Can you work these out from the model? Positions are in its coordinate system, mm. Coordinates: 2 decimals unless noted, no trailing zeros. Order: outer loops, then holes, each group sorted by start corner. A loop starts at its lowest first (then second) coordinate and runs counter-clockwise, first axis right, second up. Notation, with made-up numbers: (-8.75, -30) -> (27.25, -30) arc R37 ccw to (27.25, 6) -> close; hole circle Ø5 at (38.25, 78). An arc over 180 degrees is marked (long way). Return JSON: item names as keys, results as strings. Group by question number.
1) If we section it at A-A, the plane y = 0: Please give me the cut outline in (x, z).
2) If I drill on probe 1 along Y at (x, z) = (0, 105); probe 2 along Y at (x, z) = (6, 127); probe 3 along X at (y, z) = (7.5, 106.5), over which ranges is the centre line in solid material (lowest first)? Write a range as from..to.
3) For pin 1 (3 mm diameter, centred on x = 0.5, z = 111.5, fed in from -Y); pin 2 (1.1 mm diameter, centred on x = -0.5, z = 114, fed in from +Y); pin 3 (3 mm diameter, centred on y = -0.5, z = 75.5, fed in from -X), each with a flat end and sliding along its axis, tell me the tip position at first contact or that it passes through.
Autodesk Inventor part; units mm, degrees
ref_plane "Start Plane" through (0, 0, 10.031) normal (0, 0, 1) x (1, 0, 0)
ref_plane "End Plane" through (0, 0, 150) normal (0, 0, 1) x (1, 0, 0)
ref_plane "Work Plane6" through (-400, 9, 10.031) normal (0, 0, -1) x (-1, 0, 0)
ref_plane "Start Plane" through (0, 0, 10.031) normal (0, 0, 1) x (1, 0, 0)
ref_plane "End Plane" through (0, 0, 150) normal (0, 0, 1) x (1, 0, 0)
sketch "Sketch" plane through (0, 0, 0) normal (0, 0, 1) x (1, 0, 0)
  line L0 (0, 0) -> (2.5, 0) construction
  line L1 (0, 0) -> (0, 2.5) construction
  line L2 (0, 4) -> (0, -4) construction
  line L3 (0, 4) -> (1.7574, 4)
  arc A0 (1.7574, 4) -> (3.1716, 4.5858) centre (1.7574, 6) ccw
  line L4 (3.1716, 4.5858) -> (5.7322, 7.1464)
  line L5 (-4, 0) -> (4, 0) construction
  line L6 (4, 0) -> (4, 1.7574)
  arc A1 (4.5858, 3.1716) -> (4, 1.7574) centre (6, 1.7574) ccw
  line L7 (4.5858, 3.1716) -> (7.1464, 5.7322)
  line L8 (0, 0) -> (10, 10) construction
  line L9 (0, 0) -> (19.6827, 0) construction
  arc A2 (8, 5.3787) -> (7.1464, 5.7322) centre (7.5, 5.3787) ccw
  line L10 (8, 5.3787) -> (8, 3.5)
  arc A3 (8, 3.5) -> (8.5, 3) centre (8.5, 3.5) ccw
  line L11 (8.5, 3) -> (9.5, 3)
  arc A4 (9.5, 3) -> (10, 3.5) centre (9.5, 3.5) ccw
  line L12 (10, 3.5) -> (10, 9)
  line L13 (10, 9) -> (10, 10) construction
  arc A5 (5.7322, 7.1464) -> (5.3787, 8) centre (5.3787, 7.5) ccw
  line L14 (5.3787, 8) -> (3.5, 8)
  arc A6 (3, 8.5) -> (3.5, 8) centre (3.5, 8.5) ccw
  line L15 (3, 8.5) -> (3, 9.5)
  arc A7 (3.5, 10) -> (3, 9.5) centre (3.5, 9.5) ccw
  line L16 (3.5, 10) -> (9, 10)
  arc A8 (10, 9) -> (9, 10) centre (9, 9) ccw
  line L17 (0, 4) -> (-1.7574, 4)
  arc A9 (-3.1716, 4.5858) -> (-1.7574, 4) centre (-1.7574, 6) ccw
  line L18 (-3.1716, 4.5858) -> (-5.7322, 7.1464)
  line L19 (-4, 0) -> (-4, 1.7574)
  arc A10 (-4, 1.7574) -> (-4.5858, 3.1716) centre (-6, 1.7574) ccw
  line L20 (-4.5858, 3.1716) -> (-7.1464, 5.7322)
  arc A11 (-7.1464, 5.7322) -> (-8, 5.3787) centre (-7.5, 5.3787) ccw
  line L21 (-8, 5.3787) -> (-8, 3.5)
  arc A12 (-8.5, 3) -> (-8, 3.5) centre (-8.5, 3.5) ccw
  line L22 (-8.5, 3) -> (-9.5, 3)
  arc A13 (-10, 3.5) -> (-9.5, 3) centre (-9.5, 3.5) ccw
  line L23 (-10, 3.5) -> (-10, 9)
  arc A14 (-5.3787, 8) -> (-5.7322, 7.1464) centre (-5.3787, 7.5) ccw
  line L24 (-5.3787, 8) -> (-3.5, 8)
  arc A15 (-3.5, 8) -> (-3, 8.5) centre (-3.5, 8.5) ccw
  line L25 (-3, 8.5) -> (-3, 9.5)
  arc A16 (-3, 9.5) -> (-3.5, 10) centre (-3.5, 9.5) ccw
  line L26 (-3.5, 10) -> (-9, 10)
  arc A17 (-9, 10) -> (-10, 9) centre (-9, 9) ccw
  line L27 (0, -4) -> (-1.7574, -4)
  arc A18 (-1.7574, -4) -> (-3.1716, -4.5858) centre (-1.7574, -6) ccw
  line L28 (-3.1716, -4.5858) -> (-5.7322, -7.1464)
  arc A19 (-5.7322, -7.1464) -> (-5.3787, -8) centre (-5.3787, -7.5) ccw
  line L29 (-5.3787, -8) -> (-3.5, -8)
  arc A20 (-3, -8.5) -> (-3.5, -8) centre (-3.5, -8.5) ccw
  line L30 (-3, -8.5) -> (-3, -9.5)
  arc A21 (-3.5, -10) -> (-3, -9.5) centre (-3.5, -9.5) ccw
  line L31 (-3.5, -10) -> (-9, -10)
  arc A22 (-10, -9) -> (-9, -10) centre (-9, -9) ccw
  line L32 (-10, -3.5) -> (-10, -9)
  arc A23 (-9.5, -3) -> (-10, -3.5) centre (-9.5, -3.5) ccw
  line L33 (-8.5, -3) -> (-9.5, -3)
  arc A24 (-8, -3.5) -> (-8.5, -3) centre (-8.5, -3.5) ccw
  line L34 (-8, -5.3787) -> (-8, -3.5)
  arc A25 (-8, -5.3787) -> (-7.1464, -5.7322) centre (-7.5, -5.3787) ccw
  line L35 (-4.5858, -3.1716) -> (-7.1464, -5.7322)
  arc A26 (-4.5858, -3.1716) -> (-4, -1.7574) centre (-6, -1.7574) ccw
  line L36 (-4, 0) -> (-4, -1.7574)
  line L37 (3.5, -10) -> (9, -10)
  arc A27 (9, -10) -> (10, -9) centre (9, -9) ccw
  line L38 (10, -3.5) -> (10, -9)
  arc A28 (10, -3.5) -> (9.5, -3) centre (9.5, -3.5) ccw
  line L39 (8.5, -3) -> (9.5, -3)
  arc A29 (8.5, -3) -> (8, -3.5) centre (8.5, -3.5) ccw
  line L40 (8, -5.3787) -> (8, -3.5)
  arc A30 (7.1464, -5.7322) -> (8, -5.3787) centre (7.5, -5.3787) ccw
  line L41 (4.5858, -3.1716) -> (7.1464, -5.7322)
  arc A31 (4, -1.7574) -> (4.5858, -3.1716) centre (6, -1.7574) ccw
  line L42 (4, 0) -> (4, -1.7574)
  line L43 (5.3787, -8) -> (3.5, -8)
  arc A32 (5.3787, -8) -> (5.7322, -7.1464) centre (5.3787, -7.5) ccw
  line L44 (3.1716, -4.5858) -> (5.7322, -7.1464)
  arc A33 (3.1716, -4.5858) -> (1.7574, -4) centre (1.7574, -6) ccw
  line L45 (0, -4) -> (1.7574, -4)
  arc A34 (3.5, -8) -> (3, -8.5) centre (3.5, -8.5) ccw
  line L46 (3, -8.5) -> (3, -9.5)
  arc A35 (3, -9.5) -> (3.5, -10) centre (3.5, -9.5) ccw
  circle A36 centre (0, 0) radius 2.5
  dimension "d1" = 8
  dimension "d2" = 2
  dimension "d3" = 8
  dimension "d4" = 2
  dimension "d5" = 2
  dimension "d7" = 45
  dimension "d8" = 0.5
  dimension "d9" = 0.5
  dimension "d10" = 0.5
  dimension "d12" = 2
  dimension "d17" = 7
  dimension "d18" = 10
  dimension "d19" = 0.5
  dimension "d20" = 1
  dimension "d21" = 0.5
  dimension "d22" = 0.5
  dimension "d23" = 2
  dimension "d24" = 7
  dimension "d25" = 5
extrude "Body" add sketch "Sketch" along normal up to surface (139.969 mm away) from surface at 10.031
sketch "Sketch6" plane through (0, 0, 0) normal (0, 0, 1) x (1, 0, 0)
  line L0 (0, 0) -> (10, 0)
ref_plane "Work Plane5" through (0, 0, 0) normal (0, -1, 0) x (1, 0, 0)
sketch "Sketch7" plane through (0, 0, 0) normal (0, -1, 0) x (1, 0, 0)
  line L0 (-2, 10.031) -> (12, 10.031)
  line L1 (-2, 150) -> (12, 150)
  dimension "d33" = 139.969
ref_plane "Work Plane6" through (-400, 9, 10.031) normal (0, 0, -1) x (-1, 0, 0)
split "Split1" plane through (-400, 9, 10.031) removes the side toward (0, 0, -1)
equation "\"d1\" = 0.8 * sigma"
equation "\"d2\" = 0.2 * sigma"
equation "\"d3\" = 0.8 * sigma"
equation "\"d4\" = 0.2 * sigma"
equation "\"d5\" = 0.2 * sigma"
equation "\"d8\" = 0.05 * sigma"
equation "\"d9\" = 0.05 * sigma"
equation "\"d10\" = 0.05 * sigma"
equation "\"d12\" = 0.2 * sigma"
equation "\"d17\" = 0.7 * sigma"
equation "\"d18\" = sigma"
equation "\"d19\" = 0.05 * sigma"
equation "\"d20\" = 0.1 * sigma"
equation "\"d21\" = 0.05 * sigma"
equation "\"d22\" = 0.05 * sigma"
equation "\"d23\" = 0.2 * sigma"
equation "\"d24\" = 0.7 * sigma"
equation "\"d25\" = 0.5 * sigma"
equation "\"sigma\" = 1"
equation "\"G_OFFSET_START\" = -10.031"
equation "\"G_OFFSET_END\" = 0"
equation "\"d28\" = -G_OFFSET_START"
equation "\"G_L\" = d33"
properties part number "A3.3-MEM"
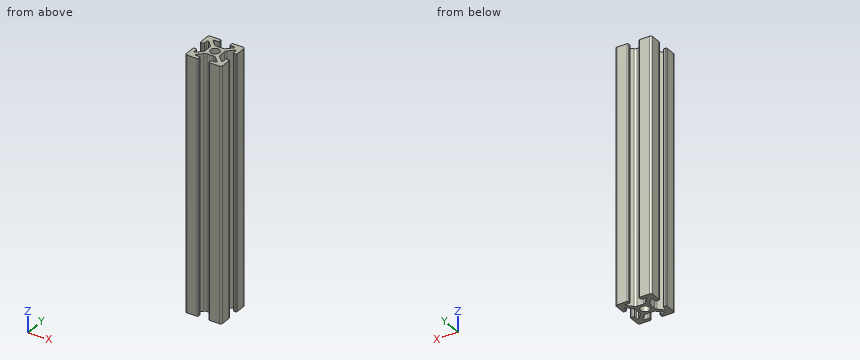
Result sheet:
{
 "1": {"outline": "(-4, 10.03) -> (-2.5, 10.03) -> (-2.5, 150) -> (-4, 150) -> close; (2.5, 10.03) -> (4, 10.03) -> (4, 150) -> (2.5, 150) -> close"},
 "2": {"probe 1": "y = -4..-2.5, 2.5..4", "probe 2": "y = -10..-4.59, 4.59..10", "probe 3": "x = -10..-5.88, 5.88..10"},
 "3": {"pin 1": "stops at y = -4.01", "pin 2": "stops at y = 4", "pin 3": "stops at x = -4.01"}
}
